from build123d import *

# Parameters (mm, degrees)
F0_W     = 25.4
F0_H     = 77.787526
F0_R     = 2.15265
F0_W_2   = 20.6375
F0_H_2   = 61.912526
F1_DEPTH = 3.175
F2_SIZE  = 3.96875


with BuildPart() as f1:
    # F0 (on Top) → F1 (new body)
    with BuildSketch(Plane.XY):
        Rectangle(F0_W, F0_H)
        with Locations((0, -34.925013)):
            Circle(F0_R, mode=Mode.SUBTRACT)
        Rectangle(F0_W_2, F0_H_2, mode=Mode.SUBTRACT)
        with Locations((0, 34.925013)):
            Circle(F0_R, mode=Mode.SUBTRACT)
    extrude(amount=F1_DEPTH)

    # F2
    f2_edges = [f1.edges().sort_by_distance(p)[0] for p in [
        (-12.7, -38.893763, 1.5875),
        (12.7, -38.893763, 1.5875),
        (12.7, 38.893763, 1.5875),
        (-12.7, 38.893763, 1.5875),
    ]]
    chamfer(f2_edges, length=F2_SIZE)


solid = f1.part
Verification items for the finished model (mm, model axes). A direction names the side the tool comes from. Coordinates: 2 decimals unless noted, no trailing zeros. Order: outer loops, then holes, each group sorted by start corner. A loop starts at its lowest first (then second) coordinate and runs counter-clockwise, first axis right, second up.
1. Go/stop test with a flat-tipped pin: pin 1 Ø4 at (x, y) = (0, -34.93) entering from -Z. Record where the tip stops, or that it passes through.
Results found:
pin 1: passes through
2. Sectioned sample at B-B, the plane x = 0. Record the cut outline in (y, z) (3 decimals).
Results found:
outline: (-38.894, 0) - (-37.078, 0) - (-37.078, 3.175) - (-38.894, 3.175) - close; (-32.772, 0) - (-30.956, 0) - (-30.956, 3.175) - (-32.772, 3.175) - close; (30.956, 0) - (32.772, 0) - (32.772, 3.175) - (30.956, 3.175) - close; (37.078, 0) - (38.894, 0) - (38.894, 3.175) - (37.078, 3.175) - close
3. Sectioned sample at D-D, the plane z = 0.8. Record the cut outline in (x, y), and give its area (3 significant figures).
Results found:
outline: (-12.7, -34.93) - (-8.73, -38.89) - (8.73, -38.89) - (12.7, -34.93) - (12.7, 34.93) - (8.73, 38.89) - (-8.73, 38.89) - (-12.7, 34.93) - close; hole (-10.32, -30.96) - (10.32, -30.96) - (10.32, 30.96) - (-10.32, 30.96) - close; hole circle Ø4.31 at (0, -34.93); hole circle Ø4.31 at (0, 34.93)
area: 637 mm2
4. Set-up check for faces 1 (the face through (10.743, 36.882, 1.565)), 2 (the face through (0, 30.956, 2)): record each of +Z, -Z, +X, -X, +Y, -Y from which the full face is reachable in a straight line by a thin tool's end or side.
Results found:
face 1: +Z, -Z, +X, +Y
face 2: +Z, -Z
5. Scan lines: line 1 (Y direction, x = 0, z = 1); line 2 (X direction, y = 13.5, z = 1.05); line 3 (Y direction, x = 1.75, z = 3). Record each from-to range of solid material in increasing order.
Results found:
line 1: y = -38.89 to -37.08, -32.77 to -30.96, 30.96 to 32.77, 37.08 to 38.89
line 2: x = -12.7 to -10.32, 10.32 to 12.7
line 3: y = -38.89 to -36.18, -33.67 to -30.96, 30.96 to 33.67, 36.18 to 38.89
6. Sectioned sample at A-A, the plane y = 26.5. Record the cut outline in (x, z) (3 decimals), and give its area (3 significant figures).
Results found:
outline: (-12.7, 0) - (-10.319, 0) - (-10.319, 3.175) - (-12.7, 3.175) - close; (10.319, 0) - (12.7, 0) - (12.7, 3.175) - (10.319, 3.175) - close
area: 15.1 mm2
7. Sectioned sample at C-C, the plane x = 3. Record the cut outline in (y, z) (3 decimals), and give its area (3 significant figures).
Results found:
outline: (-38.894, 0) - (-30.956, 0) - (-30.956, 3.175) - (-38.894, 3.175) - close; (30.956, 0) - (38.894, 0) - (38.894, 3.175) - (30.956, 3.175) - close
area: 50.4 mm2
8. Release check for a two-part mould opening along Y. For faces 3 (the face through (-12.7, 0, 2)), 4 (the face through (10.743, -36.882, 1.565)), 5 (the face through (10.319, 0, 2)) record: +Y half, -Y half, draft (parallel to the pull), parting line (faces both ways), or undercut.
Results found:
face 3: draft
face 4: -Y half
face 5: undercut
